from build123d import *

# Parameters (mm, degrees)
SKETCH_1_R          = 15
SKETCH_1_R_2        = 2
EXTRUDE_1_DEPTH     = 6
FILLET_1_R          = 3
SKETCH_3_R          = 9.5
CUT_EXTRUDE_2_DEPTH = 6
SKETCH_4_R          = 3.5
CUT_EXTRUDE_3_DEPTH = 3.5
EXTRUDE_START       = -1
SKETCH_6_R          = 9.5
SKETCH_6_R_2        = 8
EXTRUDE_3_DEPTH     = 1


with BuildPart() as part:
    # 草图1 → 凸台-拉伸1 (new body)
    with BuildSketch(Plane.XY):
        with BuildLine():
            Line((-23.911674205, 2.057142857), (-15.798784742, 96.359183673))
            ThreePointArc((-15.798784742, 96.359183673), (0, 110.857142857), (15.798784742, 96.359183673))
            Line((15.798784742, 96.359183673), (23.911674205, 2.057142857))
            ThreePointArc((23.911674205, 2.057142857), (0, -24), (-23.911674205, 2.057142857))
        make_face()
        Circle(SKETCH_1_R, mode=Mode.SUBTRACT)
        with Locations((0, 20)):
            Circle(SKETCH_1_R_2, mode=Mode.SUBTRACT)
        with Locations((17.320508076, -10)):
            Circle(SKETCH_1_R_2, mode=Mode.SUBTRACT)
        with Locations((-17.320508076, -10)):
            Circle(SKETCH_1_R_2, mode=Mode.SUBTRACT)
        with BuildLine():
            Line((-14.294598475, 20.510106154), (-9.061440494, 81.338924272))
            ThreePointArc((-9.061440494, 81.338924272), (0, 78.606870528), (9.061440494, 81.338924272))
            Line((9.061440494, 81.338924272), (14.294598475, 20.510106154))
            ThreePointArc((14.294598475, 20.510106154), (0, 25), (-14.294598475, 20.510106154))
        make_face(mode=Mode.SUBTRACT)
    extrude(amount=EXTRUDE_1_DEPTH)

    # 圆角1
    fillet_1_edges = [part.edges().sort_by_distance(p)[0] for p in [
        (-14.294598475, 20.510106154, 3),
        (14.294598475, 20.510106154, 3),
        (9.061440494, 81.338924272, 3),
        (-9.061440494, 81.338924272, 3),
    ]]
    fillet(fillet_1_edges, radius=FILLET_1_R)

    # 草图3 → 切除-拉伸2 (cut)
    with BuildSketch(Plane(origin=(0, 0, 0), x_dir=(-1, 0, 0), z_dir=(0, 0, -1))):
        with Locations((0, 95)):
            Circle(SKETCH_3_R)
    extrude(amount=-CUT_EXTRUDE_2_DEPTH, mode=Mode.SUBTRACT)

    # 草图4 → 切除-拉伸3 (cut)
    with BuildSketch(Plane.XY.offset(6)):
        with Locations((0, 20)):
            Circle(SKETCH_4_R)
        with Locations((17.320508076, -10)):
            Circle(SKETCH_4_R)
        with Locations((-17.320508076, -10)):
            Circle(SKETCH_4_R)
    extrude(amount=-CUT_EXTRUDE_3_DEPTH, mode=Mode.SUBTRACT)

    # 草图6 → 凸台-拉伸3 (add)
    with BuildSketch(Plane.XY.offset(6).offset(EXTRUDE_START)):
        with Locations(Location((0, 95, 0), (0, 0, 180))):
            Circle(SKETCH_6_R)
        with Locations((0, 95)):
            Circle(SKETCH_6_R_2, mode=Mode.SUBTRACT)
    extrude(amount=EXTRUDE_3_DEPTH)


solid = part.part
Input: part model. Units: mm. Frame: model coordinates. A direction names the side the tool comes from. Give positions to 0.01 mm unless a question says otherwise; leave off trailing zeros. Write each loop counter-clockwise with the first axis right and the second up, starting at its lowest first coordinate (ties: lowest second). Pieces come first, ordered by that corner, then holes. Notation, with made-up numbers: M 74,19 L 82,19 A16 ccw 82,45 Z; hole C 14,-24 d4. An arc over 180 degrees is marked long. Use one line per item in the form item = value.
1. Mould query, pull axis X, two halves, no side actions, for faces 6 (the face through (-0.33, 110.854, 2.958)), 7 (the face through (12.628, 23.423, 3.042)), 8 (the face through (-16, 29, 0)). Classes: released by +X, released by -X, zero draft, split by the parting line, or undercut.
Outcome:
face_6 = split by the parting line
face_7 = undercut
face_8 = zero draft
2. Cut plane B-B on z = 3.7. Return loops of the section in (x, y), and give its area (3 significant figures).
Outcome:
outline = M -23.91,2.06 A24 ccw long 23.91,2.06 L 15.8,96.36 A15.86 ccw -15.8,96.36 Z; hole C -17.32,-10 d7; hole C 0,0 d30; hole M -13.82,26.08 A3 ccw -9.67,23.06 A25 cw 9.67,23.06 A3 ccw 13.82,26.08 L 9.44,76.97 A3 ccw 5.45,79.54 A16.39 cw -5.45,79.54 A3 ccw -9.44,76.97 Z; hole C 0,95 d19; hole C 0,20 d7; hole C 17.32,-10 d7
area = 2,720 mm²
3. Cut plane C-C on x = 0. Return loops of the section in (y, z), and give its area (3 significant figures).
Outcome:
outline = M -24,0 L -15,0 L -15,6 L -24,6 Z; M 15,0 L 18,0 L 18,2.5 L 16.5,2.5 L 16.5,6 L 15,6 Z; M 22,0 L 25,0 L 25,6 L 23.5,6 L 23.5,2.5 L 22,2.5 Z; M 78.61,0 L 85.5,0 L 85.5,5 L 87,5 L 87,6 L 78.61,6 Z; M 103,5 L 104.5,5 L 104.5,0 L 110.86,0 L 110.86,6 L 103,6 Z
area = 162 mm²
4. Ray query, L1, parallel to Y at x = 0, z = 4.3; L2, parallel to Y at x = 0, z = 2.1; L3, parallel to X at y = -10, z = 1.1. Return the intervals inside material, ascending.
Outcome:
L1 = -24 to -15, 15 to 16.5, 23.5 to 25, 78.61 to 85.5, 104.5 to 110.86
L2 = -24 to -15, 15 to 18, 22 to 25, 78.61 to 85.5, 104.5 to 110.86
L3 = -21.82 to -19.32, -15.32 to -11.18, 11.18 to 15.32, 19.32 to 21.82
5. Cut plane A-A on y = 0. Return loops of the section in (x, z), and give its area (3 significant figures).
Outcome:
outline = M -24,0 L -15,0 L -15,6 L -24,6 Z; M 15,0 L 24,0 L 24,6 L 15,6 Z
area = 108 mm²
6. Cut plane D-D on x = -18. Return loops of the section in (y, z), and give its area (3 significant figures).
Outcome:
outline = M -15.87,0 L -11.88,0 L -11.88,2.5 L -13.43,2.5 L -13.43,6 L -15.87,6 Z; M -8.12,0 L 70.77,0 L 70.77,6 L -6.57,6 L -6.57,2.5 L -8.12,2.5 Z
area = 486 mm²
7. Reachability of faces 1 (the face through (1.24, 104.42, 2.46)), 2 (the face through (-20.817, -9.846, 4.274)), 3 (the face through (16, 42, 6)), 4 (the face through (8.043, 79.252, 3.042)), 5 (the face through (-19.91, 48.55, 2.96)) from +Z, -Z, +X, -X, +Y, -Y: full face, straight path, thin tool, end or side. Return the list, or none.
Outcome:
face_1 = -Z
face_2 = +Z
face_3 = +Z, +X, -X, +Y, -Y
face_4 = +Z, -Z
face_5 = +Z, -Z, -X, +Y
8. First-contact query: P1, Ø3.5, axis at x = -1.5, y = 20.5, coming from the +Z side; P2, Ø1, axis at x = -5, z = 4.5, coming from the -Y side; P3, Ø1.5, axis at x = -7, z = 2.5, coming from the -Y side. Flat tips, straight axial feed; report the tip coordinate or a pass-through.
Outcome:
P1 = 2.5
P2 = -23.57
P3 = -23.17
